Geometry: final body of the model. Coordinates: model frame, mm. Give positions to 0.01 mm unless a question says otherwise; leave off trailing zeros. Write each loop counter-clockwise with the first axis right and the second up, starting at its lowest first coordinate (ties: lowest second). Pieces come first, ordered by that corner, then holes. Notation, with made-up numbers: M -9,-33 L 27,-33 A18 cw 27,-23 Z; hole C 52.5,75 d10. An arc over 180 degrees is marked long. Use a Markdown table: item, result. Add a question column.
(1) Material intervals for L1, parallel to X at y = -23, z = -0.15; L2, parallel to Z at x = -65.25, y = 1; L3, parallel to Y at x = -60.5, z = 1.4, sorted ascending.
(2) Pin query (flat end, axial travel): pin 1 Ø0.5 at (x, y) = (-65, -26.5) entering from +Z; pin 2 Ø1.1 at (y, z) = (-10.5, -0.5) entering from -X; pin 3 Ø0.5 at (y, z) = (12.5, -0.5) entering from +X. Return the tip coordinate at first contact, or that it passes through.
(3) Cut plane B-B (z = 0.6). Output: boundary loops of the cut face in (x, y), plus the area to 3 significant figures.
(4) Cut plane A-A (y = 21). Output: boundary loops of the cut face in (x, z), plus the area to 3 significant figures.
```python
from build123d import *

# Parameters (mm, degrees)
CYLINDER003_R     = 4.85
CYLINDER003_DEPTH = 1.2
SKETCH037_W       = 1.5
SKETCH037_H       = 109
PAD020_DEPTH      = 1
BOX001_W          = 5
BOX001_H          = 5
BOX001_DEPTH      = 1.5


with BuildPart() as part:
    # Cylinder003 → Cylinder003 (join)
    with BuildSketch(Plane(origin=(0, 54.5, 0), x_dir=(1, 0, 0), z_dir=(0, 0, 1))):
        Circle(CYLINDER003_R)
    extrude(amount=CYLINDER003_DEPTH)

    # Sketch037 → Pad020 (join)
    with BuildSketch(Plane.XY):
        with Locations((-3.25, 0)):
            Rectangle(SKETCH037_W, SKETCH037_H)
        with Locations((3.25, 0)):
            Rectangle(SKETCH037_W, SKETCH037_H)
        Rectangle(SKETCH037_W, SKETCH037_H)
    extrude(amount=-PAD020_DEPTH)

    # Box001 → Box001 (join)
    with BuildSketch(Plane(origin=(-2.5, 52, 1), x_dir=(1, 0, 0), z_dir=(0, 0, 1))):
        with Locations((2.5, 2.5)):
            Rectangle(BOX001_W, BOX001_H)
    extrude(amount=BOX001_DEPTH)


with BuildPart() as part_1:
    # Body019 placement: moved
    add(part.part.moved(Location((-62, 0, 0))))


solid = part_1.part
```
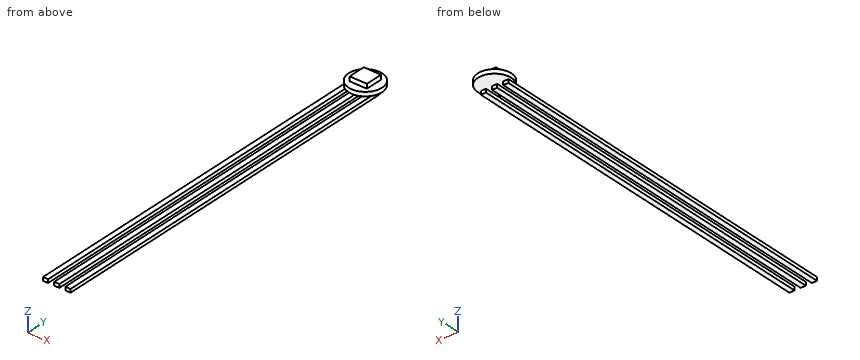
Answer list:
| question | item | result |
|---|---|---|
| 1 | L1 | -66 to -64.5, -62.75 to -61.25, -59.5 to -58 |
| 1 | L2 | -1 to 0 |
| 1 | L3 | 52 to 57 |
| 2 | pin 1 | z = 0 |
| 2 | pin 2 | x = -66 |
| 2 | pin 3 | x = -58 |
| 3 | outline | C -62,54.5 d9.7 |
| 3 | area | 73.9 mm² |
| 4 | outline | M -66,-1 L -64.5,-1 L -64.5,0 L -66,0 Z; M -62.75,-1 L -61.25,-1 L -61.25,0 L -62.75,0 Z; M -59.5,-1 L -58,-1 L -58,0 L -59.5,0 Z |
| 4 | area | 4.50 mm² |
